```python
from build123d import *

# Parameters (mm, degrees)
SKETCH1_W           = 35
SKETCH1_H           = 16
BOSS_EXTRUDE1_DEPTH = 24
SKETCH3_W           = 23.5
SKETCH3_H           = 13
CUT_EXTRUDE1_DEPTH  = 15.7
SKETCH5_R           = 0.875
CUT_EXTRUDE2_DEPTH  = 8
CUT_EXTRUDE3_REACH  = 52.513
SKETCH9_W           = 10
SKETCH9_H           = 7.5


with BuildPart() as part:
    # Sketch1 → Boss-Extrude1 (new body)
    with BuildSketch(Plane(origin=(0, 0, 0), x_dir=(1, 0, 0), z_dir=(0, 1, 0))):
        Rectangle(SKETCH1_W, SKETCH1_H)
    extrude(amount=BOSS_EXTRUDE1_DEPTH)

    # Sketch8 → Loft1 section 0
    with BuildSketch(Plane(origin=(0, 24, 0), x_dir=(1, 0, 0), z_dir=(0, 1, 0))):
        with BuildLine():
            Line((17.5, -8), (-17.5, -8))
            Line((-17.5, -8), (-17.5, 8))
            Line((-17.5, 8), (17.5, 8))
            Line((17.5, 8), (17.5, -8))
        make_face()
    # Sketch7 for Loft1 → Loft1 section 1
    with BuildSketch(Plane.XZ):
        with BuildLine():
            # circular arc as an exact rational Bezier (weights 1, cos(half-angle), 1)
            Bezier((22.73686189, 10.393994007), (0, 60.130879387), (-22.73686189, 10.393994007), weights=[1, 0.41575976, 1])
            Bezier((-22.73686189, 10.393994007), (-27.488402007, 0), (-22.73686189, -10.393994007), weights=[1, 0.909474476, 1])
            Bezier((-22.73686189, -10.393994007), (0, -60.130879387), (22.73686189, -10.393994007), weights=[1, 0.41575976, 1])
            Bezier((22.73686189, -10.393994007), (27.488402007, 0), (22.73686189, 10.393994007), weights=[1, 0.909474476, 1])
        make_face()
    loft()

    # Sketch3 → Cut-Extrude1 (cut)
    with BuildSketch(Plane.XZ.offset(-24)):
        Rectangle(SKETCH3_W, SKETCH3_H)
    extrude(amount=CUT_EXTRUDE1_DEPTH, mode=Mode.SUBTRACT)

    # Sketch5 → Cut-Extrude2 (cut)
    with BuildSketch(Plane(origin=(0, 24, 0), x_dir=(1, 0, 0), z_dir=(0, 1, 0))):
        with Locations(Location((13.2, 0, 0), (0, 0, 270))):
            Circle(SKETCH5_R)
        with Locations(Location((-14.6, 0, 0), (0, 0, 270))):
            Circle(SKETCH5_R)
    extrude(amount=-CUT_EXTRUDE2_DEPTH, mode=Mode.SUBTRACT)

    # Sketch9 → Cut-Extrude3 (cut, up to next)
    with BuildSketch(Plane.ZY.offset(-11.75), mode=Mode.PRIVATE) as cut_extrude3_sk1:
        with Locations((0, 13.7)):
            Rectangle(SKETCH9_W, SKETCH9_H)
    cut_extrude3_tool1 = extrude(cut_extrude3_sk1.sketch, amount=-CUT_EXTRUDE3_REACH, mode=Mode.PRIVATE) & part.part
    add(cut_extrude3_tool1.solids().sort_by_distance((11.75, 13.7, 0))[0], mode=Mode.SUBTRACT)


solid = part.part
```
Check sheet for the modelled part. Datum: model origin and axes. Units: mm. A direction names the side the tool comes from. Round coordinates to 2 decimals unless told otherwise and drop trailing zeros. Answer as CSV lines item,"result". Start each with the question number.
1) Tool access check on faces 1 (the face through (17, 9.95, 0)), 2 (the face through (-4, 24, 7)), 3 (the face through (-11.75, 16, 0)). Record the directions out of +Z, -Z, +X, -X, +Y, -Y that give a thin tool (end or side, any length) a straight path to the whole face; none if there is none.
2) Scan lines: probe 1 along Y at (x, z) = (13, 3.5); probe 2 along X at (y, z) = (22, 0) (3 decimals); probe 3 along Z at (x, y) = (-7.5, 10.75). Record each from-to range of solid material in increasing order.
3) Depth check by flat-ended pin: pin 1 (12 mm diameter, centred on x = -19.5, y = 7.5, fed in from -Z); pin 2 (4 mm diameter, centred on x = -0.5, z = -13.5, fed in from +Y); pin 3 (3 mm diameter, centred on y = 6, z = 3, fed in from +X). Enter the tip coordinate at first touch or a pass-through.
4) Draft check along Z on faces 4 (the face through (17, 14, -5)), 5 (the face through (-2, 0, 0)). Enter one of: +Z half, -Z half, draft (parallel to the pull), parting line (faces both ways), or undercut.
5) Section check A-A (z = 0). Give the number of separate pieces and of enclosed holes in the cut face, then the cut area to 3 significant figures.
Determined:
1,face 1,"+X"
1,face 2,"+Z, -Z, +X, -X, +Y"
1,face 3,"+Y"
2,probe 1,"0 to 9.95, 17.45 to 24"
2,probe 2,"-18.125 to -15.475, -13.725 to -11.75, 11.75 to 12.325, 14.075 to 18.125"
2,probe 3,"-16.39 to -6.5, 6.5 to 16.39"
3,pin 1,"z = -17.63"
3,pin 2,"y = 19.06"
3,pin 3,"x = 23.46"
4,face 4,"undercut"
4,face 5,"draft"
5,separate pieces,"3"
5,enclosed holes,"0"
5,area,"558 mm^2"
